```python
from build123d import *

# Parameters (mm, degrees)
CUT_EXTRUDE1_DEPTH      = 124.33016533
CUT_EXTRUDE1_DEPTH_BACK = 124.33016533


with BuildPart() as part:
    # Sketch1 → Revolve1 (revolve)
    with BuildSketch(Plane(origin=(0, 0, 0), x_dir=(1, 0, 0), z_dir=(0, 1, 0))):
        Polygon((123, 0.053684898), (-123, 0.053684898), (-123, 3.053684898), (-110, 3.053684898), (-110, 4.553684898), (-92, 4.553684898), (-92, 5.003684898), (-89.076146667, 5.003684898), (-89.076146667, 4.853684898), (-88.076146667, 4.853684898), (-88.076146667, 5.003684898), (-79.976146667, 5.003684898), (-79.976146667, 6.403684898), (79.976146667, 6.403684898), (79.976146667, 5.003684898), (88.076146667, 5.003684898), (88.076146667, 4.853684898), (89.076146667, 4.853684898), (89.076146667, 5.003684898), (92, 5.003684898), (92, 4.553684898), (110, 4.553684898), (110, 3.053684898), (123, 3.053684898), align=None)
    revolve(axis=Axis((123, 0, -0.053684898), (-1, 0, 0)))

    # Sketch5 → Cut-Extrude1 (cut, two sides: drawn at the far end of the back side and taken through both)
    with BuildSketch(Plane(origin=(0, 0, 0), x_dir=(1, 0, 0), z_dir=(0, 1, 0)).offset(-CUT_EXTRUDE1_DEPTH_BACK)):
        Polygon((-10.654863746, 304.833987592), (-10.654863746, 6.403684898), (-10.654863746, 5.35), (-20.654863746, 5.35), (-20.654863746, 6.403684898), (-20.654863746, 304.833987592), (-20.654863746, 901.69459298), (-10.654863746, 901.69459298), align=None)
    extrude(amount=CUT_EXTRUDE1_DEPTH + CUT_EXTRUDE1_DEPTH_BACK, mode=Mode.SUBTRACT)


solid = part.part
```
Geometry: final body of the model. Coordinates: model frame, mm. A direction names the side the tool comes from. Coordinates: 2 decimals unless noted, no trailing zeros. Loops run counter-clockwise (first coordinate to the right, second up) from the corner with the lowest first, then second, coordinate; pieces in that order, holes last. Notation, with made-up numbers: (8.5, 62) -> (30.5, 62) arc R16 ccw to (30.5, 72) -> close; hole circle Ø1 at (40.25, 71). An arc over 180 degrees is marked (long way). Use a Markdown table: item, result. Add a question column.
(1) Section query A-A, the plane x = -29.5. Return loops of the section in (y, z).
(2) Access query for faces 4 (the cylindrical face through (-90.518, -1.487, -4.775)), 5 (the cylindrical face through (84.083, -1.487, -4.775)), 6 (the cylindrical face through (-88.57, -4.05, -2.63)). Directions: +Z, -Z, +X, -X, +Y, -Y. A direction counts if a zero-diameter tool reaches every point of the face in a straight line with its end or side. Return the directions, or none.
(3) Mould query, pull axis X, two halves, no side actions, for faces 1 (the flat face through (-16, 0, -5.35)), 2 (the cylindrical face through (116.591, 1.825, 2.327)), 3 (the flat face through (123, 0, 0)). Classes: pulls with the +X half, pulls with the -X half, needs draft (parallel to the pull), parting line crosses it, or undercut.
(4) Section query B-B, the plane x = 85.5. Return loops of the section in (y, z).
(5) Line query: line 1 along X through (y, z) = (-4.75, -0.25); line 2 along Z through (x, y) = (-22, 4.5); line 3 along X through (y, z) = (4.25, 4.5). Output: solid intervals per line, ascending.
(6) Pin query (flat end, axial travel): pin 1 Ø4 at (x, z) = (-47.5, -4) entering from +Y; pin 2 Ø1 at (x, y) = (-68.5, 1.5) entering from +Z; pin 3 Ø1.2 at (y, z) = (1.5, -6) entering from -X. Return the tip coordinate at first contact, or that it passes through.
Answer:
| question | item | result |
|---|---|---|
| 1 | outline | circle Ø12.7 at (0, -0.05) |
| 2 | face 4 | -X |
| 2 | face 5 | +X |
| 2 | face 6 | none |
| 3 | face 1 | undercut |
| 3 | face 2 | needs draft |
| 3 | face 3 | pulls with the +X half |
| 4 | outline | circle Ø9.9 at (0, -0.05) |
| 5 | line 1 | x = -92 to 92 |
| 5 | line 2 | z = -4.53 to 4.43 |
| 5 | line 3 | x = -79.98 to 79.98 |
| 6 | pin 1 | stops at y = 6.04 |
| 6 | pin 2 | stops at z = 6.22 |
| 6 | pin 3 | stops at x = -79.98 |
